from build123d import *

# Parameters (mm, degrees)
IZIM1_W                     = 60
IZIM1_H                     = 80
Y_KSEKLIK_EKSTR_ZYON1_DEPTH = 10
IZIM2_W                     = 5
IZIM2_H                     = 19
Y_KSEKLIK_EKSTR_ZYON2_DEPTH = 50
IZIM3_W                     = 15
IZIM3_H                     = 80
Y_KSEKLIK_EKSTR_ZYON3_DEPTH = 2
Y_KSEKLIK_EKSTR_ZYON4_DEPTH = 1


with BuildPart() as part:
    # Çizim1 → Yükseklik-Ekstrüzyon1 (new body)
    with BuildSketch(Plane.XY):
        Rectangle(IZIM1_W, IZIM1_H)
    extrude(amount=Y_KSEKLIK_EKSTR_ZYON1_DEPTH)

    # Çizim2 → Yükseklik-Ekstrüzyon2 (add)
    with BuildSketch(Plane(origin=(-30, 0, 0), x_dir=(0, 0, -1), z_dir=(1, 0, 0))):
        with Locations((-2.5, 0)):
            Rectangle(IZIM2_W, IZIM2_H)
    extrude(amount=-Y_KSEKLIK_EKSTR_ZYON2_DEPTH)

    # Çizim3 → Yükseklik-Ekstrüzyon3 (add)
    with BuildSketch(Plane(origin=(30, 0, 0), x_dir=(0, 0, -1), z_dir=(1, 0, 0))):
        with Locations((-17.5, 0)):
            Rectangle(IZIM3_W, IZIM3_H)
    extrude(amount=-Y_KSEKLIK_EKSTR_ZYON3_DEPTH)

    # Çizim4 → Yükseklik-Ekstrüzyon4 (add)
    # profile 1 of 6: a face of its own
    with BuildSketch(Plane.XY.offset(10)):
        with BuildLine():
            Line((-30, -2.758821569), (-30, -22.5))
            ThreePointArc((-30, -22.5), (-20.644812954, -13.276725535), (-16.127578533, -0.940481791))
            ThreePointArc((-16.127578533, -0.940481791), (-24.247174638, 7.178595313), (-30, -2.758821569))
        make_face()
    # profile 2 of 6: a face of its own
    with BuildSketch(Plane.XY.offset(10)):
        Polygon((-21.999298336, 19.525), (-20.413706389, 19.525), (-16.567071773, 10), (-18.393078384, 10), (-19.133402903, 11.953846154), (-23.283417927, 11.953846154), (-24.023742447, 10), (-25.847841004, 10), align=None)
        Polygon((-21.207456389, 16.970117188), (-22.634679947, 13.663461538), (-19.780232831, 13.663461538), align=None, mode=Mode.SUBTRACT)
    # profile 3 of 6: a face of its own
    with BuildSketch(Plane.XY.offset(10)):
        with BuildLine():
            Line((-15.16274485, 19.525), (-13.008553144, 19.525))
            add(Edge.make_bspline(
                [(-13.008553144, 19.525), (-12.840609123, 19.523826014), (-12.515971431, 19.521556685), (-12.04563564, 19.49598681), (-11.608283206, 19.456662156), (-11.203632202, 19.402563969), (-10.832512229, 19.330977253), (-10.495401839, 19.241185748), (-10.191169607, 19.137536394), (-9.916479691, 19.015571895), (-9.665714218, 18.873373403), (-9.427604398, 18.714975699), (-9.202617755, 18.534576213), (-8.987596956, 18.335655209), (-8.78531689, 18.11457349), (-8.592408871, 17.874992969), (-8.41359616, 17.613439399), (-8.243473638, 17.336184009), (-8.089620454, 17.042051817), (-7.955423958, 16.733546416), (-7.843006739, 16.412653152), (-7.751661928, 16.079030037), (-7.678849571, 15.733784598), (-7.627904232, 15.376220162), (-7.596409316, 15.006667774), (-7.59321442, 14.756203976), (-7.591591004, 14.628936298)],
                knots=[0, 0, 0, 0, 1.44355588, 2.790409838, 4.047694926, 5.217575253, 6.298404546, 7.294384826, 8.214239204, 9.058592145, 9.873746385, 10.689560431, 11.514393297, 12.350027578, 13.205127629, 14.088021785, 14.991911688, 15.926770944, 16.882954281, 17.842803888, 18.816321264, 19.80318086, 20.814351908, 21.847355356, 22.906180909, 24, 24, 24, 24], degree=3))
            add(Edge.make_bspline(
                [(-7.591591004, 14.628936298), (-7.595841984, 14.449353321), (-7.604210287, 14.095833719), (-7.674700195, 13.577047775), (-7.788706245, 13.079739705), (-7.949009105, 12.607799646), (-8.14774174, 12.165430293), (-8.385150126, 11.760432644), (-8.657753303, 11.394980521), (-8.962375429, 11.070893577), (-9.292207001, 10.792336456), (-9.634968515, 10.553772666), (-9.993999093, 10.365645212), (-10.310355209, 10.246344273), (-10.584675428, 10.172149411), (-10.825525613, 10.128299533), (-11.099106848, 10.08808655), (-11.407970042, 10.057010822), (-11.750760277, 10.029298909), (-12.12884392, 10.014241334), (-12.540996845, 10.001730724), (-12.827276021, 10.000592025), (-12.976116245, 10)],
                knots=[0, 0, 0, 0, 1.315458931, 2.589557908, 3.828601765, 5.048913369, 6.235739168, 7.376350998, 8.481830359, 9.569842114, 10.627874879, 11.640079404, 12.624025415, 13.590060155, 14.111227486, 14.704434459, 15.382649715, 16.137166398, 16.978595427, 17.902333227, 18.909396075, 20, 20, 20, 20], degree=3))
            Line((-12.976116245, 10), (-15.16274485, 10))
            Line((-15.16274485, 10), (-15.16274485, 19.525))
        make_face()
        with BuildLine():
            Line((-13.453129466, 17.815384615), (-13.453129466, 11.709615385))
            Line((-13.453129466, 11.709615385), (-12.560160716, 11.709615385))
            add(Edge.make_bspline(
                [(-12.560160716, 11.709615385), (-12.453911148, 11.709810078), (-12.24955786, 11.710184538), (-11.954517968, 11.728020382), (-11.681680879, 11.745922652), (-11.431797647, 11.779901759), (-11.203049701, 11.817752093), (-10.998579438, 11.870426015), (-10.814171838, 11.925755509), (-10.652079405, 11.996196811), (-10.503615942, 12.075483186), (-10.366155734, 12.168376365), (-10.233468148, 12.271530737), (-10.108033884, 12.387980219), (-9.989378205, 12.516182801), (-9.878203152, 12.656799054), (-9.773024833, 12.809399953), (-9.676542976, 12.974792337), (-9.588377338, 13.151229626), (-9.510164538, 13.337002767), (-9.445314586, 13.53365885), (-9.391415276, 13.739356938), (-9.352898107, 13.955887866), (-9.321032497, 14.181647819), (-9.304604846, 14.41753124), (-9.302350253, 14.578034203), (-9.301206389, 14.659465144)],
                knots=[0, 0, 0, 0, 1.50275155, 2.890291501, 4.180787663, 5.369391935, 6.45668281, 7.458360028, 8.354766181, 9.177074746, 9.954075863, 10.732690366, 11.5210699, 12.329727389, 13.151100085, 13.990027547, 14.863562427, 15.770965086, 16.696477834, 17.652329173, 18.619756807, 19.62365428, 20.657822005, 21.729286259, 22.847956731, 24, 24, 24, 24], degree=3))
            add(Edge.make_bspline(
                [(-9.301206389, 14.659465144), (-9.303484578, 14.784250364), (-9.307926871, 15.027571875), (-9.350767379, 15.381974966), (-9.420503555, 15.715698568), (-9.520010358, 16.027504143), (-9.645441767, 16.318268029), (-9.802448416, 16.58552684), (-9.984273341, 16.833770156), (-10.12805553, 16.97939765), (-10.199899298, 17.052163462)],
                knots=[0, 0, 0, 0, 1.13821349, 2.219428113, 3.251817212, 4.244760574, 5.201143372, 6.134805572, 7.068016741, 8, 8, 8, 8], degree=3))
            add(Edge.make_bspline(
                [(-10.199899298, 17.052163462), (-10.270744054, 17.11416977), (-10.415436449, 17.240810634), (-10.669468745, 17.392558776), (-10.949399178, 17.525884392), (-11.261631718, 17.631596738), (-11.603148776, 17.715198567), (-11.975984434, 17.772856704), (-12.378142077, 17.809907212), (-12.656747521, 17.813519698), (-12.800575379, 17.815384615)],
                knots=[0, 0, 0, 0, 0.813307809, 1.661089106, 2.549956539, 3.493439533, 4.508053171, 5.589449661, 6.755572447, 8, 8, 8, 8], degree=3))
            Line((-12.800575379, 17.815384615), (-13.453129466, 17.815384615))
        make_face(mode=Mode.SUBTRACT)
    # profile 4 of 6: a face of its own
    with BuildSketch(Plane.XY.offset(10)):
        Polygon((-2.949298336, 19.525), (-1.363706389, 19.525), (2.482928227, 10), (0.656921616, 10), (-0.083402903, 11.953846154), (-4.233417927, 11.953846154), (-4.973742447, 10), (-6.797841004, 10), align=None)
        Polygon((-2.157456389, 16.970117188), (-3.584679947, 13.663461538), (-0.730232831, 13.663461538), align=None, mode=Mode.SUBTRACT)
    # profile 5 of 6: a face of its own
    with BuildSketch(Plane.XY.offset(10)):
        Polygon((3.88725515, 19.525), (5.427053827, 19.525), (9.748793611, 13.257046274), (9.748793611, 19.525), (11.458408996, 19.525), (11.458408996, 10), (9.907162001, 10), (5.596870534, 16.248873197), (5.596870534, 10), (3.88725515, 10), align=None)
    # profile 6 of 6: a face of its own
    with BuildSketch(Plane.XY.offset(10)):
        Polygon((16.589163202, 19.525), (18.17475515, 19.525), (22.021389765, 10), (20.195383154, 10), (19.455058635, 11.953846154), (15.305043611, 11.953846154), (14.564719092, 10), (12.740620534, 10), align=None)
        Polygon((17.38100515, 16.970117188), (15.953781592, 13.663461538), (18.808228707, 13.663461538), align=None, mode=Mode.SUBTRACT)
    extrude(amount=Y_KSEKLIK_EKSTR_ZYON4_DEPTH)


solid = part.part
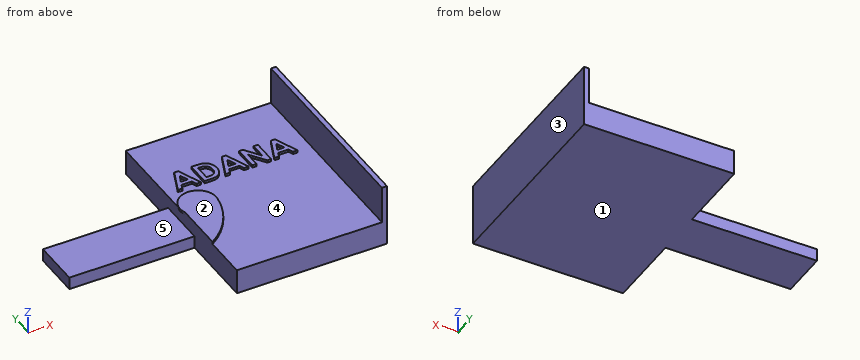
Part model, mm, in its own coordinate system. Face numbers are marked on the shaded views. A direction names the side the tool comes from. Give positions to 0.01 mm unless a question says otherwise; leave off trailing zeros. Loops run counter-clockwise (first coordinate to the right, second up) from the corner with the lowest first, then second, coordinate; pieces in that order, holes last.
(1) Band-saw the part on D-D (y = -5). Write the cut outline in (x, z).
Return value:
outline: (-80, 0) - (30, 0) - (30, 25) - (28, 25) - (28, 10) - (-16.95, 10) - (-16.95, 11) - (-30, 11) - (-30, 5) - (-80, 5) - close
(2) Pin check, flat tips, straight feed: pin 1 (4 mm diameter, centred on x = -44, z = 2, fed in from -Y); pin 2 (1.5 mm diameter, centred on y = 1, z = 19, fed in from -X); pin 3 (0.5 mm diameter, centred on x = -13.5, z = 10.5, fed in from -Y). Stop position of each tip, or through.
Return value:
pin 1: stops at y = -9.5
pin 2: stops at x = 28
pin 3: stops at y = 10
(3) Drill centre lines: line 1 along Y through (x, z) = (-55, 4.5); line 2 along Z through (x, y) = (-29.5, 22); line 3 along Z through (x, y) = (-55.5, -1). Where is each one in solid material? Low to high.
Return value:
line 1: y = -9.5 to 9.5
line 2: z = 0 to 10
line 3: z = 0 to 5
(4) 3-axis set-ups, long thin cutter, end or side, ignore diameter. For the marked faces 1 and 2: which of +Z, -Z, +X, -X, +Y, -Y reach the whole face in a straight line?
Return value:
face 1: -Z, +X, -X, +Y, -Y
face 2: +Z, -X, +Y, -Y
(5) Band-saw the part on A-A (y = 21.5). Write the cut outline in (x, z), and give its area (3 significant figures).
Return value:
outline: (-30, 0) - (30, 0) - (30, 25) - (28, 25) - (28, 10) - (-30, 10) - close
area: 630 mm2
(6) Band-saw the part on C-C (z = 20). Write the cut outline in (x, y), and give its area (3 significant figures).
Return value:
outline: (28, -40) - (30, -40) - (30, 40) - (28, 40) - close
area: 160 mm2
(7) Pull direction X, two halves, no side cores. Call the marked faces 3, 4 and 5: pulls with the +X half, pulls with the -X half, needs draft (parallel to the pull), parting line crosses it, or undercut.
Return value:
face 3: pulls with the +X half
face 4: undercut
face 5: needs draft
(8) Band-saw the part on B-B (x = -41.5). Write the cut outline in (y, z).
Return value:
outline: (-9.5, 0) - (9.5, 0) - (9.5, 5) - (-9.5, 5) - close
